Source: CAD feature listing. Evaluate the final solid. Frame: model axes, mm. A direction names the side the tool comes from. Give positions to 0.01 mm unless a question says otherwise; leave off trailing zeros. Order: outer loops, then holes, each group sorted by start corner. A loop starts at its lowest first (then second) coordinate and runs counter-clockwise, first axis right, second up. Notation, with made-up numbers: (65, 4.25) - (72, 4.25) arc R6 ccw to (72, 10.25) - close; hole circle Ø2 at (63, 26.5). An arc over 180 degrees is marked (long way). Use CSV: the item, a comma, the result in double quotes.
```python
from build123d import *

# Parameters (mm, degrees)
BOSS_EXTRUDE1_DEPTH  = 10
CUT_EXTRUDE1_DEPTH   = 79.460180984
FILLET1_R            = 6
FILLET4_R            = 3
FILLET5_R            = 10
FILLET1_OF_MIRROR2_R = 6
FILLET4_OF_MIRROR2_R = 3
FILLET5_OF_MIRROR2_R = 10
CUT_EXTRUDE2_DEPTH   = 2
SKETCH4_W            = 7.3
SKETCH4_H            = 3.5
CUT_EXTRUDE3_DEPTH   = 79.230429006


with BuildPart() as part:
    # Sketch1 → Boss-Extrude1 (new body)
    with BuildSketch(Plane.XY):
        with BuildLine():
            Line((-70, 16.58258549), (-70, 2.58258549))
            Line((-70, 2.58258549), (-65, -0.035347018))
            ThreePointArc((-65, -0.035347018), (-62.639321295, -11.428715409), (-59.057390955, -22.499009997))
            ThreePointArc((-59.057390955, -22.499009997), (-50.858075368, -30.911196539), (-39.524366721, -34))
            Line((-39.524366721, -34), (-29.119439011, -34))
            ThreePointArc((-29.119439011, -34), (-16.364659062, -29.873537236), (-8.443933007, -19.058075838))
            ThreePointArc((-8.443933007, -19.058075838), (-5.792248942, -9.629238804), (-4, 0))
            Line((-4, 0), (0, 0))
            Line((0, 0), (0, 19))
            Line((0, 19), (-62, 19))
            Line((-62, 19), (-70, 16.58258549))
        make_face()
    boss_extrude1 = extrude(amount=BOSS_EXTRUDE1_DEPTH)

    # Sketch2 → Cut-Extrude1 (cut, through all)
    with BuildSketch(Plane.XY.offset(10)):
        with BuildLine():
            Line((-39.524366721, -29), (-29.119439011, -29))
            ThreePointArc((-29.119439011, -29), (-19.293350153, -25.821035725), (-13.191343035, -17.488968441))
            ThreePointArc((-13.191343035, -17.488968441), (-10.661621804, -8.493805879), (-8.951806424, 0.692541077))
            ThreePointArc((-8.951806424, 0.692541077), (-8.83111114, 2.375291538), (-8.93749946, 4.05900707))
            ThreePointArc((-8.93749946, 4.05900707), (-33.987475013, 7.999161751), (-59.288689209, 6.303681198))
            ThreePointArc((-59.288689209, 6.303681198), (-60.075532666, 3.563074376), (-60.056140486, 0.711816353))
            ThreePointArc((-60.056140486, 0.711816353), (-57.852345066, -9.972645379), (-54.521869403, -20.361214511))
            ThreePointArc((-54.521869403, -20.361214511), (-48.178176596, -26.685865227), (-39.524366721, -29))
        make_face()
    cut_extrude1 = extrude(amount=-CUT_EXTRUDE1_DEPTH, mode=Mode.SUBTRACT)

    # Fillet1
    fillet1_edges = [part.edges().sort_by_distance(p)[0] for p in [
        (-8.93749946, 4.05900707, 5),
        (-59.288689209, 6.303681198, 5),
    ]]
    fillet(fillet1_edges, radius=FILLET1_R)

    # Fillet4
    fillet4_edges = [part.edges().sort_by_distance(p)[0] for p in [
        (-4, 0, 5),
    ]]
    fillet(fillet4_edges, radius=FILLET4_R)

    # Fillet5
    fillet5_edges = [part.edges().sort_by_distance(p)[0] for p in [
        (-65, -0.035347018, 5),
        (-62, 19, 5),
    ]]
    fillet(fillet5_edges, radius=FILLET5_R)

    # Mirror2: Boss-Extrude1, Cut-Extrude1 across plane
    add(boss_extrude1.mirror(Plane(origin=(0, 19, 10), x_dir=(0, 0, 1), z_dir=(1, 0, 0))))
    add(cut_extrude1.mirror(Plane(origin=(0, 19, 10), x_dir=(0, 0, 1), z_dir=(1, 0, 0))), mode=Mode.SUBTRACT)

    # Fillet1 of Mirror2
    fillet1_of_mirror2_edges = [part.edges().sort_by_distance(p)[0] for p in [
        (8.93749946, 4.05900707, 5),
        (59.288689209, 6.303681198, 5),
    ]]
    fillet(fillet1_of_mirror2_edges, radius=FILLET1_OF_MIRROR2_R)

    # Fillet4 of Mirror2
    fillet4_of_mirror2_edges = [part.edges().sort_by_distance(p)[0] for p in [
        (4, 0, 5),
    ]]
    fillet(fillet4_of_mirror2_edges, radius=FILLET4_OF_MIRROR2_R)

    # Fillet5 of Mirror2
    fillet5_of_mirror2_edges = [part.edges().sort_by_distance(p)[0] for p in [
        (65, -0.035347018, 5),
        (62, 19, 5),
    ]]
    fillet(fillet5_of_mirror2_edges, radius=FILLET5_OF_MIRROR2_R)

    # Sketch3 → Cut-Extrude2 (cut)
    with BuildSketch(Plane.XY.offset(10)):
        Polygon((-68.579000582, 15.967320332), (-61.852211578, 18), (61.852211578, 18), (68.579000582, 15.967320332), (68.579000582, 2.967348727), (66.731457293, 2), (61.632252323, 2), (57.126911514, 9.5), (18.95111491, 9.5), (4.382114171, 2), (-4.382114171, 2), (-18.95111491, 9.5), (-57.126911514, 9.5), (-61.632252323, 2), (-66.731457293, 2), (-68.579000582, 2.967348727), align=None)
    extrude(amount=-CUT_EXTRUDE2_DEPTH, mode=Mode.SUBTRACT)

    # Sketch4 → Cut-Extrude3 (cut, through all)
    with BuildSketch(Plane.XY.offset(8)):
        with Locations((0, 14)):
            Rectangle(SKETCH4_W, SKETCH4_H)
        with Locations((0, 6.5)):
            Rectangle(SKETCH4_W, SKETCH4_H)
    extrude(amount=-CUT_EXTRUDE3_DEPTH, mode=Mode.SUBTRACT)


solid = part.part
```
Item 1: First-contact query: pin 1 (2.5 mm diameter, centred on x = -0.5, z = 3.5, fed in from -Y); pin 2 (3.5 mm diameter, centred on x = 1.5, z = 3, fed in from -Y); pin 3 (1 mm diameter, centred on y = -7.5, z = 8, fed in from +X). Flat tips, straight axial feed; report the tip coordinate or a pass-through.
Filled in:
pin 1,"stops at y = -0.02"
pin 2,"stops at y = -0.62"
pin 3,"stops at x = 63.71"
Item 2: Material intervals for line 1 (X direction, y = -13.5, z = 1); line 2 (X direction, y = -22, z = 9.5); line 3 (X direction, y = 1.5, z = 8), sorted ascending. Write a range as from..to.
Filled in:
line 1,"x = -62.07..-56.86, -11.96..-6.77, 6.77..11.96, 56.86..62.07"
line 2,"x = -59.25..-53.44, -15.49..-9.66, 9.66..15.49, 53.44..59.25"
line 3,"x = -68.15..-60.02, -9.57..9.57, 60.02..68.15"
Item 3: Section C-C on z = 3.5. Count the separate pieces of the cut face and the enclosed holes in it, then the cut area to 3 significant figures.
Filled in:
separate pieces,"1"
enclosed holes,"4"
area,"2,850 mm2"
Item 4: Set-up query: faces 4 (the flat face through (59.41, 5.7, 9.01)), 5 (the flat face through (3.65, 6, 4)), 6 (the flat face through (0, 0, 5)). Return all of +Z, -Z, +X, -X, +Y, -Y with unobstructed straight access to the full face (end or side cutting, diameter ignored); none if empty.
Filled in:
face 4,"+Z"
face 5,"+Z, -Z"
face 6,"+Z, -Z, -Y"
Item 5: Section B-B on x = 31. Return the cut outline in (y, z).
Filled in:
outline,"(-34, 0) - (-29, 0) - (-29, 10) - (-34, 10) - close; (7.83, 0) - (19, 0) - (19, 10) - (18, 10) - (18, 8) - (9.5, 8) - (9.5, 10) - (7.83, 10) - close"
Item 6: Section A-A on y = -11.5. Return the cut outline in (x, z).
Filled in:
outline,"(-62.62, 0) - (-57.44, 0) - (-57.44, 10) - (-62.62, 10) - close; (-11.41, 0) - (-6.25, 0) - (-6.25, 10) - (-11.41, 10) - close; (6.25, 0) - (11.41, 0) - (11.41, 10) - (6.25, 10) - close; (57.44, 0) - (62.62, 0) - (62.62, 10) - (57.44, 10) - close"
Item 7: Section D-D on x = 47.5. Return the cut outline in (y, z).
Filled in:
outline,"(-32.53, 0) - (-27.06, 0) - (-27.06, 10) - (-32.53, 10) - close; (7.8, 0) - (19, 0) - (19, 10) - (18, 10) - (18, 8) - (9.5, 8) - (9.5, 10) - (7.8, 10) - close"
Item 8: Mould query, pull axis Y, two halves, no side actions, for faces 1 (the cylindrical face through (-66.03, -0.576, 5.07)), 2 (the flat face through (-66.66, 17.59, 4.93)), 3 (the cylindrical face through (10.95, -9.69, 5.07)). Classes: released by +Y, released by -Y, zero draft, split by the parting line, or undercut.
Filled in:
face 1,"released by -Y"
face 2,"released by +Y"
face 3,"undercut"
